Geometry: final body of the model. Coordinates: model frame, mm. Round coordinates to 2 decimals unless told otherwise and drop trailing zeros. Order: outer loops, then holes, each group sorted by start corner. A loop starts at its lowest first (then second) coordinate and runs counter-clockwise, first axis right, second up. Notation, with made-up numbers: M 39.5,4.5 L 85.5,4.5 A33 ccw 85.5,42.5 Z; hole C 46.25,-8 d7. An arc over 180 degrees is marked long. Return JSON: item names as keys, results as strings. Group by question number.
Q1. Contact query for flat-ended pins moving along their axis: pin 1 (1.5 mm diameter, centred on y = -5.5, z = -19, fed in from -X); pin 2 (1 mm diameter, centred on x = 1.5, z = -23.5, fed in from +Y); pin 3 (10 mm diameter, centred on y = 4, z = -26, fed in from +X); pin 4 (1 mm diameter, centred on x = -8.5, z = -52, fed in from -Y). Output: stop coordinate, or through.
Q2. Cut plane C-C on y = 3.5. Output: boundary loops of the cut face in (x, z).
Q3. Cut plane B-B on x = 8.25. Output: boundary loops of the cut face in (y, z).
Q4. Ray query, probe 1 along Y at (x, z) = (1.75, -76.5); probe 2 along Y at (x, z) = (-9.5, -55); probe 3 along X at (y, z) = (1.5, -78.5). Return the intervals inside material, ascending.
Q5. Cut plane A-A on z = -34. Output: boundary loops of the cut face in (x, y) (3 decimals).
```python
from build123d import *

# Parameters (mm, degrees)
F1_DEPTH    = 9.525
F0_W        = 23.402531108
F0_H        = 85.8396906406
F3_T1_DEPTH = 136.6396906406
F4_R        = 5.08


# Not quite as in the source:
# - a fillet or chamfer that OpenCascade refuses, or shapes differently, is made with other operations: its cross-section is extruded or revolved along the edge and cut away or added


with BuildPart() as f1:
    # F0 (on Front) → F1 (new body, symmetric)
    with BuildSketch(Plane.XZ):
        Polygon((-2.3270829115, -113.9840111136), (-12.9329506308, -113.9840111136), (-12.9329506308, -186.3234937191), (-2.3270829115, -199.3203783987), (8.2787848078, -186.3234937191), (8.2787848078, -113.9840111136), align=None)
    extrude(amount=F1_DEPTH, both=True)


with BuildPart() as f1b:
    # F0 (on Front) → F1, piece 2 (new body, symmetric)
    with BuildSketch(Plane.XZ):
        with Locations((-1.2316850768, -52.651762031)):
            Rectangle(F0_W, F0_H)
    extrude(amount=F1_DEPTH, both=True)

    # F3: fillet of radius 10.16 on 2 edges, made by hand

    # F3_s2 → F3_t1 (cut)
    with BuildSketch(Plane.XY.offset(-120.9716073513)):
        with BuildLine():
            ThreePointArc((0.3095804772, -9.525), (7.4937853741, -6.5492048969), (10.4695804772, 0.635))
            Line((10.4695804772, 0.635), (10.4695804772, -9.525))
            Line((10.4695804772, -9.525), (0.3095804772, -9.525))
        make_face()
        with BuildLine():
            ThreePointArc((10.4695804772, -0.635), (7.4937853741, 6.5492048969), (0.3095804772, 9.525))
            Line((0.3095804772, 9.525), (10.4695804772, 9.525))
            Line((10.4695804772, 9.525), (10.4695804772, -0.635))
        make_face()
    extrude(amount=F3_T1_DEPTH, mode=Mode.SUBTRACT)

    # F4
    f4_edges = [f1b.edges().sort_by_distance(p)[0] for p in [
        (-12.932951, 9.525, -52.651762),
        (-12.932951, -9.525, -52.651762),
    ]]
    fillet(f4_edges, radius=F4_R)


solid = f1b.part
```
Result sheet:
{
 "1": {"pin 1": "stops at x = -12.92", "pin 2": "stops at y = 9.5", "pin 3": "stops at x = 10.45", "pin 4": "stops at y = -9.52"},
 "2": {"outline": "M -12.93,-95.57 L 9.59,-95.57 L 9.59,-9.73 L -12.93,-9.73 Z"},
 "3": {"outline": "M -5.7,-95.57 L 5.7,-95.57 L 5.7,-9.73 L -5.7,-9.73 Z"},
 "4": {"probe 1": "y = -9.42 to 9.42", "probe 2": "y = -9.25 to 9.25", "probe 3": "x = -12.93 to 10.24"},
 "5": {"outline": "M -12.933,-4.445 A5.08 ccw -7.853,-9.525 L 0.31,-9.525 A10.16 ccw 10.45,0 A10.16 ccw 0.31,9.525 L -7.853,9.525 A5.08 ccw -12.933,4.445 Z"}
}
